Geometry check sheet. Reference: the model listing, model coordinates, mm. Face numbers are marked on the shaded views. A direction names the side the tool comes from. Round coordinates to 2 decimals unless told otherwise and drop trailing zeros. Order: outer loops, then holes, each group sorted by start corner. A loop starts at its lowest first (then second) coordinate and runs counter-clockwise, first axis right, second up. Notation, with made-up numbers: (27, 49) - (51, 49) arc R12 ccw to (51, 64) - close; hole circle Ø11 at (-26.5, 1.25). An arc over 180 degrees is marked (long way). Use a Markdown table: item, result. Add a question column.
(1) Gauge pin test, flat ends, axial feed: P1, Ø2.5, axis at x = 44.4, z = 0, coming from the -Y side; P2, Ø1.5, axis at x = 19.5, y = 1.5, coming from the -Z side; P3, Ø1, axis at x = 2, z = 1, coming from the -Y side. Record the tip position at first contact, or that the pin passes through.
(2) Access from +Z, -Z, +X, -X, +Y, -Y to the whole of each face (thin tool, end or side, straight path). Record for the marked faces 1, 2 and 3.
(3) Section check B-B on x = -16. Record the boundary of the cut face in (y, z).
(4) Thickness scan on line 1 along X through (y, z) = (-0.75, 4.75); line 2 along X through (y, z) = (-1.3, 0); line 3 along Y through (x, z) = (1, 0.25). Record the ranges inside material, lowest first. Write a range as [from, to].
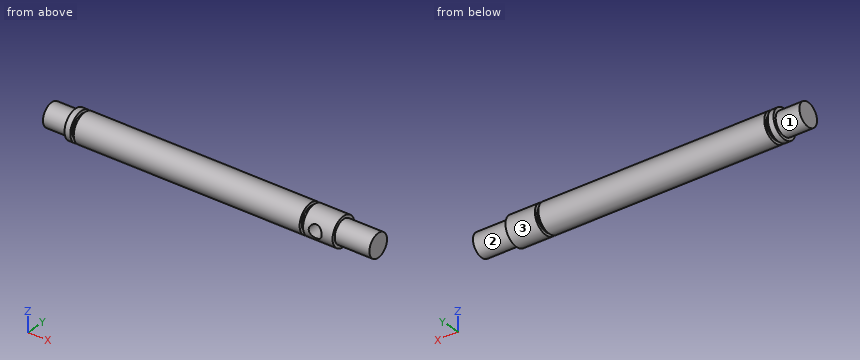
```python
from build123d import *

# Parameters (mm, degrees)
M4_CLEARANCE_HOLE5_D     = 4.5
M4_CLEARANCE_HOLE5_DEPTH = 5.1
M4_CLEARANCE_HOLE5_TIP   = 1.351936393
SKETCH17_R               = 4
BOSS_EXTRUDE1_DEPTH      = 12


with BuildPart() as part:
    # Sketch1 → Revolve1 (revolve)
    with BuildSketch(Plane.XY):
        Polygon((-39.2, -5), (39, -5), (39, -4), (40.2, -4), (40.2, -5), (50.4, -5), (50.4, 0), (-50.6, 0), (-50.6, -4), (-42.4, -4), (-42.4, -5), (-40.4, -5), (-40.4, -4), (-39.2, -4), align=None)
    revolve(axis=Axis((0, 0, 0), (1, 0, 0)))

    # M4 Clearance Hole5
    with Locations(Plane(origin=(44.4, -5, 0), x_dir=(0, 0, -1), z_dir=(0, -1, 0))):
        with Locations((0, 0)):
            Hole(M4_CLEARANCE_HOLE5_D / 2, depth=M4_CLEARANCE_HOLE5_DEPTH)
            with Locations((0, 0, -(M4_CLEARANCE_HOLE5_DEPTH + M4_CLEARANCE_HOLE5_TIP / 2))):  # 118° drill point
                Cone(0, M4_CLEARANCE_HOLE5_D / 2, M4_CLEARANCE_HOLE5_TIP, mode=Mode.SUBTRACT)

    # Sketch17 → Boss-Extrude1 (add)
    with BuildSketch(Plane(origin=(50.4, 0, 0), x_dir=(0, 0, -1), z_dir=(1, 0, 0))):
        Circle(SKETCH17_R)
    extrude(amount=BOSS_EXTRUDE1_DEPTH)


solid = part.part
```
Check sheet entries:
| question | item | result |
|---|---|---|
| 1 | P1 | stops at y = 0.7 |
| 1 | P2 | stops at z = -4.94 |
| 1 | P3 | stops at y = -4.97 |
| 2 | face 1 | -X |
| 2 | face 2 | +X |
| 2 | face 3 | +X, -X |
| 3 | outline | circle Ø10 at (0, 0) |
| 4 | line 1 | x = [-42.4, -40.4], [-39.2, 39], [40.2, 50.4] |
| 4 | line 2 | x = [-50.6, 42.15], [46.65, 62.4] |
| 4 | line 3 | y = [-4.99, 4.99] |
